Part print with two shaded views. Sizes in mm from the minimum x, y, z corner. A direction names the side the tool comes from. Give positions to 0.01 mm unless a question says otherwise; leave off trailing zeros. Write each loop counter-clockwise with the first axis right and the second up, starting at its lowest first coordinate (ties: lowest second). Pieces come first, ordered by that corner, then holes. Notation, with made-up numbers: (47.25, -26) -> (99.25, -26) arc R14 cw to (99.25, -15) -> close; hole circle Ø6 at (32, 78.25). An arc over 180 degrees is marked (long way). Answer as a JSON object with one key per item and string values.
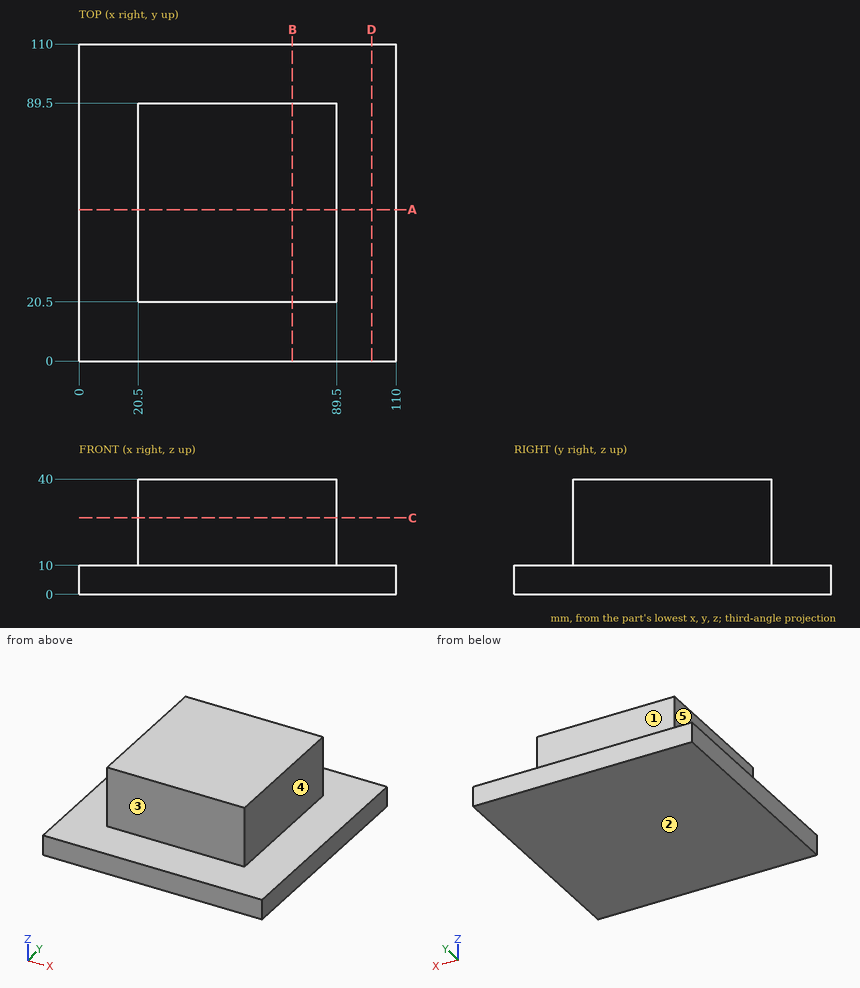
1) Wall check: probe 1 along X at (y, z) = (28, 28); probe 2 along Z at (x, y) = (52, 99). Give the ranges that are in metal, low to high.
Model answer:
{"probe 1": "x = 20.5 to 89.5", "probe 2": "z = 0 to 10"}
2) Slice it at D-D (x = 101.5). List the corners of the cut face in (y, z).
Model answer:
{"outline": "(0, 0) -> (110, 0) -> (110, 10) -> (0, 10) -> close"}
3) Pin check, flat tips, straight feed: pin 1 (10 mm diameter, centred on x = 69.5, z = 24.5, fed in from -Y); pin 2 (10 mm diameter, centred on y = 27, z = 26.5, fed in from +X); pin 3 (2 mm diameter, centred on x = 22.5, z = 21, fed in from +Y); pin 4 (10 mm diameter, centred on y = 12, z = 25.5, fed in from -X). Stop position of each tip, or through.
Model answer:
{"pin 1": "stops at y = 20.5", "pin 2": "stops at x = 89.5", "pin 3": "stops at y = 89.5", "pin 4": "passes through"}
4) 3-axis set-ups, long thin cutter, end or side, ignore diameter. For the marked faces 1, 2, 3, 4 and 5: which of +Z, -Z, +X, -X, +Y, -Y reach the whole face in a straight line?
Model answer:
{"face 1": "+Z, +X, -X, +Y", "face 2": "-Z, +X, -X, +Y, -Y", "face 3": "+Z, +X, -X, -Y", "face 4": "+Z, +X, +Y, -Y", "face 5": "+Z, -X, +Y, -Y"}
5) Slice it at C-C (z = 26.5). List the corners of the cut face in (x, y), then the cut area to 3 significant figures.
Model answer:
{"outline": "(20.5, 20.5) -> (89.5, 20.5) -> (89.5, 89.5) -> (20.5, 89.5) -> close", "area": "4,760 mm2"}
6) Slice it at A-A (y = 52.5). List the corners of the cut face in (x, z), then the cut area to 3 significant figures.
Model answer:
{"outline": "(0, 0) -> (110, 0) -> (110, 10) -> (89.5, 10) -> (89.5, 40) -> (20.5, 40) -> (20.5, 10) -> (0, 10) -> close", "area": "3,170 mm2"}
